Read the model definition and answer for the solid it produces. Units are mm, in the model's axes. A direction names the side the tool comes from. Give positions to 0.01 mm unless a question says otherwise; leave off trailing zeros. Write each loop counter-clockwise with the first axis right and the second up, starting at its lowest first coordinate (ties: lowest second). Pieces come first, ordered by that corner, then holes. Notation, with made-up numbers: (44.5, -13) - (65.5, -13) arc R21 ccw to (65.5, 7) - close; hole circle Ø4 at (80.5, 12.25). An arc over 180 degrees is marked (long way). Use CSV: the item, a comma, the result in double quotes. Start each with the question number.
from build123d import *

# Parameters (mm, degrees)
SKETCH_1_R          = 12.5
EXTRUDE_1_DEPTH     = 17
SKETCH_2_R          = 16
EXTRUDE_2_DEPTH     = 51
SKETCH_3_R          = 2
EXTRUDE_3_DEPTH     = 11
SKETCH_4_R          = 4
EXTRUDE_4_DEPTH     = 5
SKETCH_5_R          = 8
EXTRUDE_5_DEPTH     = 1.98
SKETCH_6_R          = 1.5
EXTRUDE_6_DEPTH     = 2
SKETCH_7_R          = 20.782497367
SKETCH_7_R_2        = 13.5
CUT_EXTRUDE_8_DEPTH = 4


with BuildPart() as part:
    # Эскиз1 → Вытянуть1 (new body)
    with BuildSketch(Plane.XY):
        Circle(SKETCH_1_R)
    extrude(amount=EXTRUDE_1_DEPTH)

    # Эскиз2 → Вытянуть2 (add)
    with BuildSketch(Plane.XY.offset(17)):
        Circle(SKETCH_2_R)
    extrude(amount=EXTRUDE_2_DEPTH)

    # Эскиз3 → Вытянуть3 (add)
    with BuildSketch(Plane.XY.offset(68)):
        Circle(SKETCH_3_R)
    extrude(amount=EXTRUDE_3_DEPTH)

    # Эскиз4 → Вытянуть4 (add)
    with BuildSketch(Plane.XY.offset(72)):
        Circle(SKETCH_4_R)
    extrude(amount=EXTRUDE_4_DEPTH)

    # Эскиз5 → Вытянуть5 (add)
    with BuildSketch(Plane.XY.offset(77)):
        Circle(SKETCH_5_R)
    extrude(amount=EXTRUDE_5_DEPTH)

    # Эскиз6 → Вытянуть6 (add)
    with BuildSketch(Plane.XY.offset(78.98)):
        with Locations((0, -6.154904873)):
            Circle(SKETCH_6_R)
        with Locations(Location((0, 6.154904873, 0), (0, 0, 180))):
            Circle(SKETCH_6_R)
    extrude(amount=EXTRUDE_6_DEPTH)

    # Эскиз7 → Вытянуть8 (cut)
    with BuildSketch(Plane.XY.offset(38)):
        Circle(SKETCH_7_R)
        Circle(SKETCH_7_R_2, mode=Mode.SUBTRACT)
    extrude(amount=CUT_EXTRUDE_8_DEPTH, mode=Mode.SUBTRACT)


solid = part.part
(1) Which of the six approach directions +Z, -Z, +X, -X, +Y, -Y give full straight-line access (tool end or side, diameter ignored) to faces 5 (the face through (0, 0, 0)), 6 (the face through (-1.73, -7.81, 77.98)), 7 (the face through (11.923, 3.755, 8.381)), 8 (the face through (-2, -1, 72))?
(2) Consider probe 1 along Z at (x, y) = (-4, -3); probe 2 along Z at (x, y) = (8, -12); probe 3 along Z at (x, y) = (-8.5, 3). Determine where each line is inside the solid, lowest interval first.
(3) The part is cut by section C-C on z = 52.5. Write down the section's boundary in (x, y), plus the area to 3 significant figures.
(4) The part is cut by section B-B on x = 11. Write down the section's boundary in (y, z).
(5) For a pull along Z with two mould halves and no side action, classify faces 1 (the face through (-3.47, -15.62, 27.35)), 2 (the face through (-10, -8, 17)), 3 (the face through (0, 6, 80.98)), 4 (the face through (-4, -2, 77)) as pulls with the +Z half, pulls with the -Z half, needs draft (parallel to the pull), parting line crosses it, or undercut.
(6) The part is cut by section D-D on y = 10. Write down the section's boundary in (x, z), plus the area to 3 significant figures.
(7) Given P1, Ø12, axis at y = -8, z = 48, coming from the +X side; P2, Ø6, axis at x = 10, y = 10, coming from the -Z side; P3, Ø9.5, axis at x = 6.5, y = -2, coming from the +Z side; P4, Ø5, axis at y = -4.5, z = 31, coming from the -X side, each flat-ended and moving along its own axis, determine where each tip first touches the part or whether it passes through.
Reported:
1,face 5,"-Z, +X, -X, +Y, -Y"
1,face 6,"+Z"
1,face 7,"-Z"
1,face 8,"none"
2,probe 1,"0 to 68, 77 to 78.98"
2,probe 2,"17 to 38, 42 to 68"
2,probe 3,"0 to 68"
3,outline,"circle Ø32 at (0, 0)"
3,area,"804 mm²"
4,outline,"(-11.62, 17) - (-5.94, 17) - (-5.94, 0) - (5.94, 0) - (5.94, 17) - (11.62, 17) - (11.62, 38) - (7.83, 38) - (7.83, 42) - (11.62, 42) - (11.62, 68) - (-11.62, 68) - (-11.62, 42) - (-7.83, 42) - (-7.83, 38) - (-11.62, 38) - close"
5,face 1,"needs draft"
5,face 2,"pulls with the -Z half"
5,face 3,"pulls with the +Z half"
5,face 4,"undercut"
6,outline,"(-12.49, 17) - (-7.5, 17) - (-7.5, 0) - (7.5, 0) - (7.5, 17) - (12.49, 17) - (12.49, 38) - (9.07, 38) - (9.07, 42) - (12.49, 42) - (12.49, 68) - (-12.49, 68) - (-12.49, 42) - (-9.07, 42) - (-9.07, 38) - (-12.49, 38) - close"
6,area,"1,500 mm²"
7,P1,"x = 15.87"
7,P2,"z = 0"
7,P3,"z = 78.98"
7,P4,"x = -15.87"
